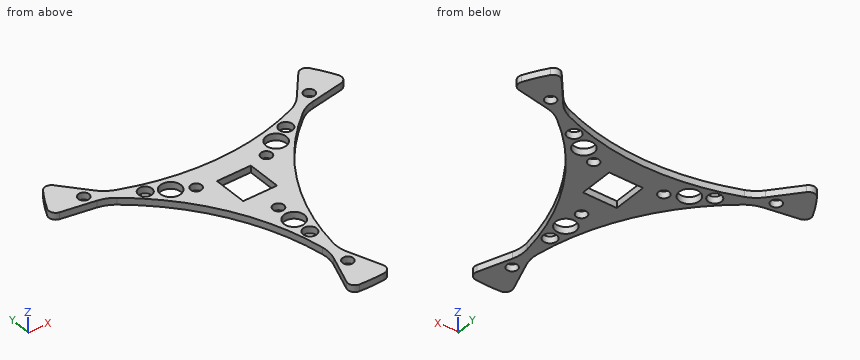
from build123d import *

# Parameters (mm, degrees)
SKETCH_1_R          = 47.75
EXTRUDE_1_DEPTH     = 2
SKETCH_2_R          = 1.6
CUT_EXTRUDE_1_DEPTH = 68.558308149
FILLET_1_R          = 10
SKETCH_3_R          = 1.6
SKETCH_3_R_2        = 3
SKETCH_3_R_3        = 2
SKETCH_3_W          = 10
SKETCH_3_H          = 10
CUT_EXTRUDE_2_DEPTH = 66.049417533
FILLET_2_R          = 2


with BuildPart() as part:
    # ｽｹｯﾁ1 → ﾎﾞｽ - 押し出し1 (new body)
    with BuildSketch(Plane.XY):
        Circle(SKETCH_1_R)
    extrude(amount=EXTRUDE_1_DEPTH)

    # ｽｹｯﾁ2 → ｶｯﾄ - 押し出し1 (cut, through all)
    with BuildSketch(Plane.XY.offset(2)):
        with Locations((0, -38.5)):
            Circle(SKETCH_2_R)
        with Locations((-33.341978046, 19.25)):
            Circle(SKETCH_2_R)
        with Locations((33.341978046, 19.25)):
            Circle(SKETCH_2_R)
        with BuildLine():
            Line((-44.128949923, 18.240018604), (-29.553612406, 15.669993347))
            ThreePointArc((-29.553612406, 15.669993347), (-10.20639232, -5.892663354), (-1.206193887, -33.429175791))
            Line((-1.206193887, -33.429175791), (-6.268155485, -47.336800978))
            ThreePointArc((-6.268155485, -47.336800978), (-41.352713031, -23.875), (-44.128949923, 18.240018604))
        make_face()
        with BuildLine():
            Line((6.268155485, -47.336800978), (1.206193887, -33.429175791))
            ThreePointArc((1.206193887, -33.429175791), (10.20639232, -5.892663354), (29.553612406, 15.669993347))
            Line((29.553612406, 15.669993347), (44.128949923, 18.240018604))
            ThreePointArc((44.128949923, 18.240018604), (41.352713031, -23.875), (6.268155485, -47.336800978))
        make_face()
        with BuildLine():
            Line((-37.860794438, 29.096782374), (-28.347418519, 17.759182444))
            ThreePointArc((-28.347418519, 17.759182444), (0, 11.785326707), (28.347418519, 17.759182444))
            Line((28.347418519, 17.759182444), (37.860794438, 29.096782374))
            ThreePointArc((37.860794438, 29.096782374), (0, 47.75), (-37.860794438, 29.096782374))
        make_face()
    extrude(amount=-CUT_EXTRUDE_1_DEPTH, mode=Mode.SUBTRACT)

    # ﾌｨﾚｯﾄ1
    fillet_1_edges = [part.edges().sort_by_distance(p)[0] for p in [
        (1.206193887, -33.429175791, 1),
        (29.553612406, 15.669993347, 1),
        (28.347418519, 17.759182444, 1),
        (-28.347418519, 17.759182444, 1),
        (-29.553612406, 15.669993347, 1),
        (-1.206193887, -33.429175791, 1),
    ]]
    fillet(fillet_1_edges, radius=FILLET_1_R)

    # ｽｹｯﾁ3 → ｶｯﾄ - 押し出し2 (cut, through all)
    with BuildSketch(Plane(origin=(0, 0, 0), x_dir=(-1, 0, 0), z_dir=(0, 0, -1))):
        with Locations((-10.392304845, 6)):
            Circle(SKETCH_3_R)
        with Locations((0, -12)):
            Circle(SKETCH_3_R)
        with Locations((10.392304845, 6)):
            Circle(SKETCH_3_R)
        with Locations((0, -18)):
            Circle(SKETCH_3_R_2)
        with Locations((0, -24)):
            Circle(SKETCH_3_R_3)
        with Locations((-15.588457268, 9)):
            Circle(SKETCH_3_R_2)
        with Locations((-20.784609691, 12)):
            Circle(SKETCH_3_R_3)
        with Locations((15.588457268, 9)):
            Circle(SKETCH_3_R_2)
        with Locations((20.784609691, 12)):
            Circle(SKETCH_3_R_3)
        Rectangle(SKETCH_3_W, SKETCH_3_H)
    extrude(amount=-CUT_EXTRUDE_2_DEPTH, mode=Mode.SUBTRACT)

    # ﾌｨﾚｯﾄ2
    fillet_2_edges = [part.edges().sort_by_distance(p)[0] for p in [
        (44.128949923, 18.240018604, 1),
        (6.268155485, -47.336800978, 1),
        (-37.860794438, 29.096782374, 1),
        (37.860794438, 29.096782374, 1),
        (-6.268155485, -47.336800978, 1),
        (-44.128949923, 18.240018604, 1),
    ]]
    fillet(fillet_2_edges, radius=FILLET_2_R)


solid = part.part
The listing builds one solid part. Answer for the finished solid, in the listing's coordinates (mm). Round coordinates to 2 decimals unless told otherwise and drop trailing zeros. Loops run counter-clockwise (first coordinate to the right, second up) from the corner with the lowest first, then second, coordinate; pieces in that order, holes last. Notation, with made-up numbers: M -35,-12 L -30,-12 A17 cw -30,-6 Z; hole C 86.25,-31 d8. An arc over 180 degrees is marked long. Write each question's results on one line, items separated by ' | '. Start each with the question number.
1) Each of these flat-tipped pins is pushed along its axis until it touches: pin 1 (3.5 mm diameter, centred on x = 0, y = -12, fed in from -Z); pin 2 (2.5 mm diameter, centred on x = 0, y = -38.5, fed in from +Z); pin 3 (1 mm diameter, centred on x = -2, z = 0.5, fed in from -Y). Where does it stop, or does it pass through?
2) Find section A-A on x = 0. Write down the section's boundary in (y, z).
3) Find section C-C on z = 1.15. Count the separate pieces of the cut face and the enclosed holes in it, plus the area to 3 significant figures.
4) Straight lines are drawn through the part: probe 1 along Y at (x, z) = (0, 0.9); probe 2 along X at (y, z) = (18, 1.2); probe 3 along Y at (x, z) = (-14, 1.4). For each, find the intervals that lie inside material, in ascending order.
Final values:
1) pin 1: z = 0 | pin 2: through | pin 3: y = -47.73
2) outline: M -47.75,0 L -40.1,0 L -40.1,2 L -47.75,2 Z; M -36.9,0 L -26,0 L -26,2 L -36.9,2 Z; M -22,0 L -21,0 L -21,2 L -22,2 Z; M -15,0 L -13.6,0 L -13.6,2 L -15,2 Z; M -10.4,0 L -5,0 L -5,2 L -10.4,2 Z; M 5,0 L 11.79,0 L 11.79,2 L 5,2 Z
3) separate pieces: 1 | enclosed holes: 13 | area: 993 mm²
4) probe 1: -47.75 to -40.1, -36.9 to -26, -22 to -21, -15 to -13.6, -10.4 to -5, 5 to 11.79 | probe 2: -42.2 to -34.34, -32.34 to -28.19, 28.19 to 32.34, 34.34 to 42.2 | probe 3: -0.02 to 6.46, 11.54 to 13.19
